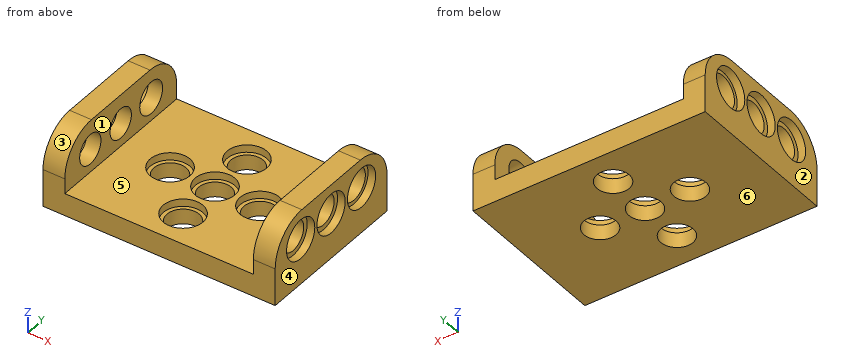
```python
from build123d import *

# Parameters (mm, degrees)
CROQUIS1_W              = 31
CROQUIS1_H              = 21
SALIENTE_EXTRUIR1_DEPTH = 10
CROQUIS2_W              = 25.17
CROQUIS2_H              = 21
CORTAR_EXTRUIR1_DEPTH   = 7
CROQUIS5_R              = 2.15
CORTAR_EXTRUIR2_DEPTH   = 11
CROQUIS6_R              = 2.15
CROQUIS6_R_2            = 2
CORTAR_EXTRUIR4_DEPTH   = 32
CROQUIS6_3_R            = 2.65
CROQUIS6_3_R_2          = 2.15
CROQUIS6_3_R_3          = 2
CORTAR_EXTRUIR5_DEPTH   = 1.015
CROQUIS9_R              = 2.65
CROQUIS9_R_2            = 2.15
CROQUIS9_R_3            = 2
CORTAR_EXTRUIR6_DEPTH   = 1.015
REDONDEO5_R             = 5
CROQUIS10_R             = 2.65
CROQUIS10_R_2           = 2.15
CORTAR_EXTRUIR8_DEPTH   = 1


with BuildPart() as part:
    # Croquis1 → Saliente-Extruir1 (new body)
    with BuildSketch(Plane.XY):
        with Locations((28.576975021, 10.857913544)):
            Rectangle(CROQUIS1_W, CROQUIS1_H)
    extrude(amount=SALIENTE_EXTRUIR1_DEPTH)

    # Croquis2 → Cortar-Extruir1 (cut)
    with BuildSketch(Plane.XY.offset(10)):
        with Locations((28.576975021, 10.857913544)):
            Rectangle(CROQUIS2_W, CROQUIS2_H)
    extrude(amount=-CORTAR_EXTRUIR1_DEPTH, mode=Mode.SUBTRACT)

    # Croquis5 → Cortar-Extruir2 (cut, through all)
    with BuildSketch(Plane(origin=(0, 0, 0), x_dir=(-1, 0, 0), z_dir=(0, 0, -1))):
        with Locations((-28.576975021, 16.857913544)):
            Circle(CROQUIS5_R)
        with Locations((-28.576975021, 10.857913544)):
            Circle(CROQUIS5_R)
        with Locations((-22.576975021, 10.857913544)):
            Circle(CROQUIS5_R)
        with Locations((-34.576975021, 10.857913544)):
            Circle(CROQUIS5_R)
        with Locations((-28.576975021, 4.857913544)):
            Circle(CROQUIS5_R)
    extrude(amount=-CORTAR_EXTRUIR2_DEPTH, mode=Mode.SUBTRACT)

    # Croquis6 → Cortar-Extruir4 (cut, through all)
    with BuildSketch(Plane(origin=(44.076975021, 0, 0), x_dir=(0, 0, -1), z_dir=(1, 0, 0))):
        with Locations((-6.107568768, 16.572862239)):
            Circle(CROQUIS6_R)
        with Locations((-6.107568768, 10.857913544)):
            Circle(CROQUIS6_R_2)
        with Locations((-6.107568768, 5.142964849)):
            Circle(CROQUIS6_R_2)
    extrude(amount=-CORTAR_EXTRUIR4_DEPTH, mode=Mode.SUBTRACT)

    # Croquis6_3 → Cortar-Extruir5 (cut)
    with BuildSketch(Plane(origin=(44.076975021, 0, 0), x_dir=(0, 0, -1), z_dir=(1, 0, 0))):
        with Locations((-6.107568768, 16.572862239)):
            Circle(CROQUIS6_3_R)
        with Locations((-6.107568768, 16.572862239)):
            Circle(CROQUIS6_3_R_2, mode=Mode.SUBTRACT)
        with Locations((-6.107568768, 10.857913544)):
            Circle(CROQUIS6_3_R)
        with Locations((-6.107568768, 10.857913544)):
            Circle(CROQUIS6_3_R_3, mode=Mode.SUBTRACT)
        with Locations((-6.107568768, 5.142964849)):
            Circle(CROQUIS6_3_R)
        with Locations((-6.107568768, 5.142964849)):
            Circle(CROQUIS6_3_R_3, mode=Mode.SUBTRACT)
    extrude(amount=-CORTAR_EXTRUIR5_DEPTH, mode=Mode.SUBTRACT)

    # Croquis9 → Cortar-Extruir6 (cut)
    with BuildSketch(Plane.ZY.offset(-13.076975021)):
        with Locations((6.107568768, 16.572862239)):
            Circle(CROQUIS9_R)
        with Locations((6.107568768, 16.572862239)):
            Circle(CROQUIS9_R_2, mode=Mode.SUBTRACT)
        with Locations((6.107568768, 10.857913544)):
            Circle(CROQUIS9_R)
        with Locations((6.107568768, 10.857913544)):
            Circle(CROQUIS9_R_3, mode=Mode.SUBTRACT)
        with Locations((6.107568768, 5.142964849)):
            Circle(CROQUIS9_R)
        with Locations((6.107568768, 5.142964849)):
            Circle(CROQUIS9_R_3, mode=Mode.SUBTRACT)
    extrude(amount=-CORTAR_EXTRUIR6_DEPTH, mode=Mode.SUBTRACT)

    # Redondeo5
    redondeo5_edges = [part.edges().sort_by_distance(p)[0] for p in [
        (42.619475021, 21.357913544, 10),
        (42.619475021, 0.357913544, 10),
        (14.534475021, 21.357913544, 10),
        (14.534475021, 0.357913544, 10),
    ]]
    fillet(redondeo5_edges, radius=REDONDEO5_R)

    # Croquis10 → Cortar-Extruir8 (cut)
    with BuildSketch(Plane.XY.offset(3)):
        with Locations((28.576975021, 16.857913544)):
            Circle(CROQUIS10_R)
        with Locations((28.576975021, 16.857913544)):
            Circle(CROQUIS10_R_2, mode=Mode.SUBTRACT)
        with Locations((34.576975021, 10.857913544)):
            Circle(CROQUIS10_R)
        with Locations((34.576975021, 10.857913544)):
            Circle(CROQUIS10_R_2, mode=Mode.SUBTRACT)
        with Locations((28.576975021, 10.857913544)):
            Circle(CROQUIS10_R)
        with Locations((28.576975021, 10.857913544)):
            Circle(CROQUIS10_R_2, mode=Mode.SUBTRACT)
        with Locations((22.576975021, 10.857913544)):
            Circle(CROQUIS10_R)
        with Locations((22.576975021, 10.857913544)):
            Circle(CROQUIS10_R_2, mode=Mode.SUBTRACT)
        with Locations((28.576975021, 4.857913544)):
            Circle(CROQUIS10_R)
        with Locations((28.576975021, 4.857913544)):
            Circle(CROQUIS10_R_2, mode=Mode.SUBTRACT)
    extrude(amount=-CORTAR_EXTRUIR8_DEPTH, mode=Mode.SUBTRACT)


solid = part.part
```
Check sheet for the modelled part. Datum: model origin and axes. Units: mm. Face numbers are marked on the shaded views. A direction names the side the tool comes from. Coordinates: 2 decimals unless noted, no trailing zeros. Order: outer loops, then holes, each group sorted by start corner. A loop starts at its lowest first (then second) coordinate and runs counter-clockwise, first axis right, second up. Notation, with made-up numbers: (-11.5, -30.75) -> (19.5, -30.75) arc R20 cw to (19.5, -0.75) -> close; hole circle Ø7 at (44.25, 35.25). An arc over 180 degrees is marked (long way). Write item = value, one per line. Start each with the question number.
1) Cross-section at B-B (x = 33). Enter the section's corners in (y, z), then the cut area to 3 significant figures.
2) Cross-section at C-C (x = 41.5). Enter the section's corners in (y, z), then the cut area to 3 significant figures.
3) Mould release check, pull along X, two halves, no side actions. Record for the marked faces 1, 2, 3 and 4: +X half, -X half, draft (parallel to the pull), parting line (faces both ways), or undercut.
4) Access from +Z, -Z, +X, -X, +Y, -Y to the whole of each face (thin tool, end or side, straight path). Record for the marked faces 5 and 6.
5) Go/stop test with flat-tipped pins: P1, Ø8, axis at x = 36, y = 13.5, coming from the +Z side; P2, Ø1.6, axis at x = 29.5, y = 18, coming from the +Z side; P3, Ø5, axis at y = 5.14, z = 6.11, coming from the -X side; P4, Ø5, axis at x = 26, z = 4.5, coming from the -Y side. Record where each tip stops, or that it passes through.
6) Material ranges on L1, parallel to X at y = 12.25, z = 8; L2, parallel to X at y = 10.75, z = 1.25; L3, parallel to X at y = 14.25, z = 4.5, recorded low to high.
7) Cross-section at D-D (x = 29.5). Enter the section's corners in (y, z), then the cut area to 3 significant figures.
8) Cross-section at A-A (y = 4.25). State how many separate pieces and enclosed holes the cut face has, then the cut area to 3 significant figures.
Ans:
q1.outline = (0.36, 0) -> (9.4, 0) -> (9.4, 2) -> (8.73, 2) -> (8.73, 3) -> (0.36, 3) -> close; (12.32, 0) -> (21.36, 0) -> (21.36, 3) -> (12.99, 3) -> (12.99, 2) -> (12.32, 2) -> close
q1.area = 52.9 mm²
q2.outline = (0.36, 0) -> (21.36, 0) -> (21.36, 5) arc R5 ccw to (16.36, 10) -> (5.36, 10) arc R5 ccw to (0.36, 5) -> close; hole circle Ø4 at (5.14, 6.11); hole circle Ø4 at (10.86, 6.11); hole circle Ø4.3 at (16.57, 6.11)
q2.area = 160 mm²
q3.face_1 = undercut
q3.face_2 = -X half
q3.face_3 = draft
q3.face_4 = +X half
q4.face_5 = +Z, +Y, -Y
q4.face_6 = -Z, +X, -X, +Y, -Y
q5.P1 = 3
q5.P2 = 2
q5.P3 = 14.09
q5.P4 = 0.36
q6.L1 = 14.09 to 15.99, 41.16 to 43.06
q6.L2 = 13.08 to 20.43, 24.72 to 26.43, 30.72 to 32.43, 36.72 to 44.08
q6.L3 = 13.08 to 15.99, 41.16 to 44.08
q7.outline = (0.36, 0) -> (2.92, 0) -> (2.92, 2) -> (2.37, 2) -> (2.37, 3) -> (0.36, 3) -> close; (6.8, 0) -> (8.92, 0) -> (8.92, 2) -> (8.37, 2) -> (8.37, 3) -> (7.34, 3) -> (7.34, 2) -> (6.8, 2) -> close; (12.8, 0) -> (14.92, 0) -> (14.92, 2) -> (14.37, 2) -> (14.37, 3) -> (13.34, 3) -> (13.34, 2) -> (12.8, 2) -> close; (18.8, 0) -> (21.36, 0) -> (21.36, 3) -> (19.34, 3) -> (19.34, 2) -> (18.8, 2) -> close
q7.area = 24.8 mm²
q8.separate_pieces = 4
q8.enclosed_holes = 0
q8.area = 95.9 mm²
